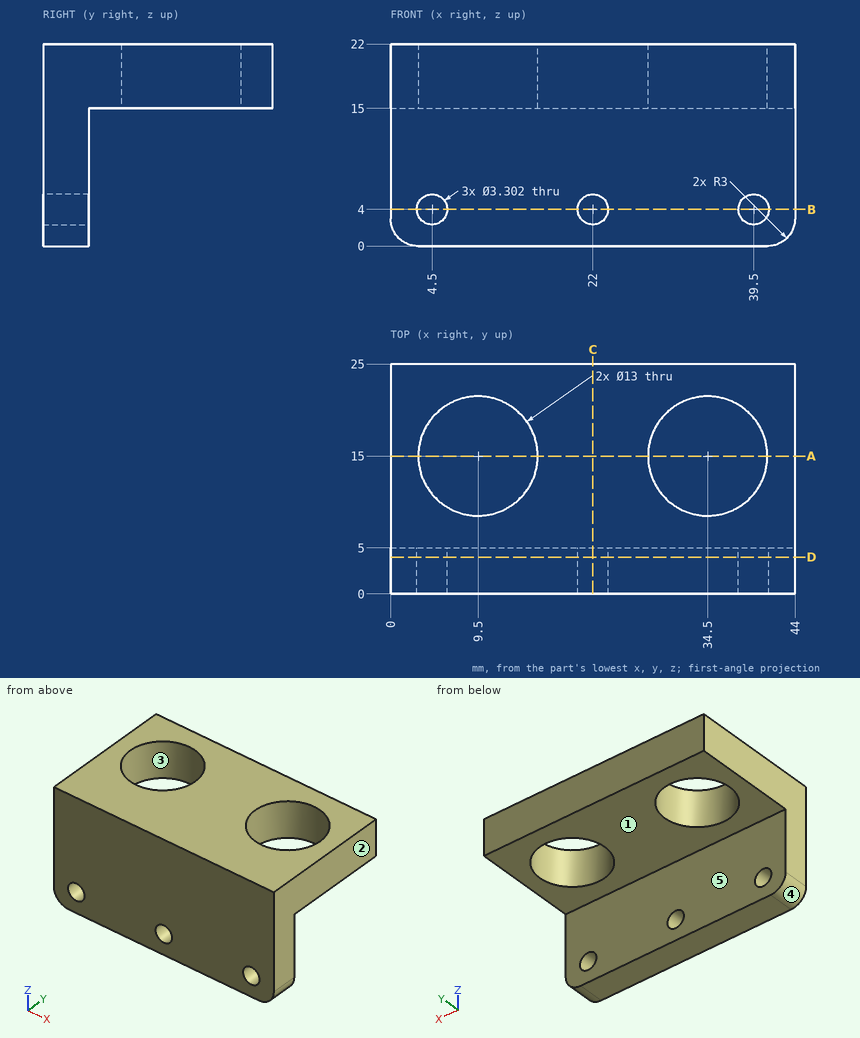
Check sheet for the drawn part. Datum: minimum x, y, z corner. Units: mm. A direction names the side the tool comes from. Coordinates: 2 decimals unless noted, no trailing zeros. Loops run counter-clockwise (first coordinate to the right, second up) from the corner with the lowest first, then second, coordinate; pieces in that order, holes last. Notation, with made-up numbers: (13, -19) -> (39, -19) arc R30 ccw to (39, 15) -> close; hole circle Ø7 at (44, 51). An arc over 180 degrees is marked (long way). Answer as CSV lines item,"result".
1) Tool access check on the marked faces 1 and 2. Record the directions out of +Z, -Z, +X, -X, +Y, -Y that give a thin tool (end or side, any length) a straight path to the whole face; none if there is none.
Found:
face 1,"-Z, +X, -X, +Y"
face 2,"+Z, -Z, +X, +Y, -Y"
2) Thickness scan on L1, parallel to X at y = 3.5, z = 4; L2, parallel to Y at x = 18.5, z = 12.5; L3, parallel to Z at x = 24.5, y = 10.5. Record the ranges inside material, lowest first. Write a range as from..to.
Found:
L1,"x = 0..2.85, 6.15..20.35, 23.65..37.85, 41.15..44"
L2,"y = 0..5"
L3,"z = 15..22"
3) Cross-section at B-B, the plane z = 4. Record the cut outline in (x, y).
Found:
outline,"(0, 0) -> (2.85, 0) -> (2.85, 5) -> (0, 5) -> close; (6.15, 0) -> (20.35, 0) -> (20.35, 5) -> (6.15, 5) -> close; (23.65, 0) -> (37.85, 0) -> (37.85, 5) -> (23.65, 5) -> close; (41.15, 0) -> (44, 0) -> (44, 5) -> (41.15, 5) -> close"
4) Cross-section at D-D, the plane y = 4. Record the cut outline in (x, z), then the cut area to 3 significant figures.
Found:
outline,"(0, 3) arc R3 ccw to (3, 0) -> (41, 0) arc R3 ccw to (44, 3) -> (44, 22) -> (0, 22) -> close; hole circle Ø3.3 at (4.5, 4); hole circle Ø3.3 at (22, 4); hole circle Ø3.3 at (39.5, 4)"
area,"938 mm2"
5) Release check for a two-part mould opening along X. For the marked faces 3, 4 and 5 record: +X half, -X half, draft (parallel to the pull), parting line (faces both ways), or undercut.
Found:
face 3,"undercut"
face 4,"-X half"
face 5,"draft"
6) Depth check by flat-ended pin: pin 1 (5.5 mm diameter, centred on x = 39.5, z = 4, fed in from +Y); pin 2 (5 mm diameter, centred on x = 10, y = 10.5, fed in from -Z). Enter the tip coordinate at first touch or a pass-through.
Found:
pin 1,"stops at y = 5"
pin 2,"stops at z = 15"
7) Cross-section at C-C, the plane x = 22. Record the cut outline in (y, z), then the cut area to 3 significant figures.
Found:
outline,"(0, 0) -> (5, 0) -> (5, 2.35) -> (0, 2.35) -> close; (0, 5.65) -> (5, 5.65) -> (5, 15) -> (25, 15) -> (25, 22) -> (0, 22) -> close"
area,"233 mm2"
8) Cross-section at A-A, the plane y = 15. Record the cut outline in (x, z), then the cut area to 3 significant figures.
Found:
outline,"(0, 15) -> (3, 15) -> (3, 22) -> (0, 22) -> close; (16, 15) -> (28, 15) -> (28, 22) -> (16, 22) -> close; (41, 15) -> (44, 15) -> (44, 22) -> (41, 22) -> close"
area,"126 mm2"
